```python
from build123d import *

# Parameters (mm, degrees)
BOX142_W     = 49.5
BOX142_H     = 2
BOX142_DEPTH = 2
BOX143_W     = 3
BOX143_H     = 15
BOX143_DEPTH = 2
BOX144_W     = 3
BOX144_H     = 15
BOX144_DEPTH = 2
BOX139_W     = 7
BOX139_H     = 15
BOX139_DEPTH = 2


with BuildPart() as cube131:
    # Box142 → Box142 (new body)
    with BuildSketch(Plane(origin=(34.5, -2, 2), x_dir=(1, 0, 0), z_dir=(0, 0, 1))):
        with Locations((24.75, 1)):
            Rectangle(BOX142_W, BOX142_H)
    extrude(amount=BOX142_DEPTH)


with BuildPart() as cube132:
    # Box143 → Box143 (new body)
    with BuildSketch(Plane(origin=(34.5, -17, 2), x_dir=(1, 0, 0), z_dir=(0, 0, 1))):
        with Locations((1.5, 7.5)):
            Rectangle(BOX143_W, BOX143_H)
    extrude(amount=BOX143_DEPTH)


with BuildPart() as cube133:
    # Box144 → Box144 (new body)
    with BuildSketch(Plane(origin=(81, -17, 2), x_dir=(1, 0, 0), z_dir=(0, 0, 1))):
        with Locations((1.5, 7.5)):
            Rectangle(BOX144_W, BOX144_H)
    extrude(amount=BOX144_DEPTH)


with BuildPart() as fusion047:
    # Box139 → Box139 (new body)
    with BuildSketch(Plane(origin=(55.5, -17, 2), x_dir=(1, 0, 0), z_dir=(0, 0, 1))):
        with Locations((3.5, 7.5)):
            Rectangle(BOX139_W, BOX139_H)
    extrude(amount=BOX139_DEPTH)

    # Fusion047: union Cube131, Cube132, Cube133
    add(cube131.part)
    add(cube132.part)
    add(cube133.part)


solid = fusion047.part
```
The listing builds one solid part. Answer for the finished solid, in the listing's coordinates (mm). A direction names the side the tool comes from. Give positions to 0.01 mm unless a question says otherwise; leave off trailing zeros. Order: outer loops, then holes, each group sorted by start corner. A loop starts at its lowest first (then second) coordinate and runs counter-clockwise, first axis right, second up. Notation, with made-up numbers: (75, 66) -> (93, 66) arc R11 cw to (93, 78) -> close; hole circle Ø6 at (7, 42.25). An arc over 180 degrees is marked (long way). Write each question's results on one line, items separated by ' | '.
Q1. The part is cut by section C-C, the plane x = 44.5. Give the vertices of the cut face in (y, z), and give its area (3 significant figures).
Checked values:
outline: (-2, 2) -> (0, 2) -> (0, 4) -> (-2, 4) -> close | area: 4.00 mm^2
Q2. Which of the six approach directions +Z, -Z, +X, -X, +Y, -Y give full straight-line access (tool end or side, diameter ignored) to faces 1 (the face through (59, 0, 3)), 2 (the face through (55.5, -10, 3))?
Checked values:
face 1: +Z, -Z, +X, -X, +Y | face 2: +Z, -Z, -Y
Q3. The part is cut by section B-B, the plane z = 3.15. Give the vertices of the cut face in (x, y).
Checked values:
outline: (34.5, -17) -> (37.5, -17) -> (37.5, -2) -> (55.5, -2) -> (55.5, -17) -> (62.5, -17) -> (62.5, -2) -> (81, -2) -> (81, -17) -> (84, -17) -> (84, 0) -> (34.5, 0) -> close
Q4. Straight lines are drawn through the part: probe 1 along X at (y, z) = (-11.75, 2.3); probe 2 along Y at (x, z) = (79.5, 3.85). For each, find the intervals that lie inside material, in ascending order. Write a range as from..to.
Checked values:
probe 1: x = 34.5..37.5, 55.5..62.5, 81..84 | probe 2: y = -2..0
Q5. The part is cut by section A-A, the plane y = -7.5. Give the vertices of the cut face in (x, z).
Checked values:
outline: (34.5, 2) -> (37.5, 2) -> (37.5, 4) -> (34.5, 4) -> close; (55.5, 2) -> (62.5, 2) -> (62.5, 4) -> (55.5, 4) -> close; (81, 2) -> (84, 2) -> (84, 4) -> (81, 4) -> close
Q6. This flat-tipped pin is pushed along its axis until it touches: P1, Ø0.6, axis at x = 46, z = 3.5, coming from the -Y side. Where does it stop, or does it pass through?
Checked values:
P1: stops at y = -2
